Model file for the job. Use its own axes, mm. Face numbers are marked on the shaded views. A direction names the side the tool comes from. Give positions to 0.01 mm unless a question says otherwise; leave off trailing zeros. Write each loop counter-clockwise with the first axis right and the second up, starting at its lowest first coordinate (ties: lowest second). Pieces come first, ordered by that corner, then holes. Notation, with made-up numbers: (87.25, 26.5) - (116.25, 26.5) arc R18 cw to (116.25, 44.5) - close; hole circle Ø9 at (27.5, -33). An arc over 180 degrees is marked (long way). Use a Markdown table: item, result. Add a question column.
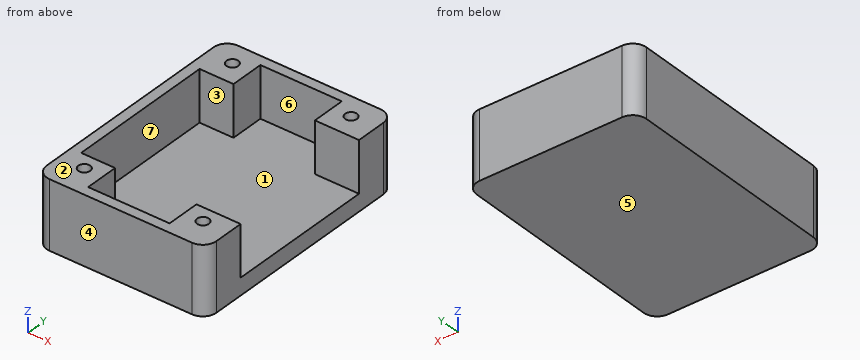
Autodesk Inventor part; units mm, degrees
ref_plane "YZ Plane" through (0, 0, 0) normal (1, 0, 0) x (0, 1, 0)
ref_plane "XZ Plane" through (0, 0, 0) normal (0, 1, 0) x (-1, 0, 0)
ref_plane "XY Plane" through (0, 0, 0) normal (0, 0, 1) x (1, 0, 0)
sketch "Sketch1" plane through (0, 0, 0) normal (0, 0, 1) x (1, 0, 0)
  line L0 (0, 0) -> (50, 0)
  line L1 (50, 0) -> (50, 70)
  line L2 (50, 70) -> (0, 70)
  line L3 (0, 70) -> (0, 0)
  dimension "d0" = 50
  dimension "d1" = 70
extrude "Extrusion1" add sketch "Sketch1" along normal blind 20
sketch "Sketch2" plane through (0, 0, 20) normal (0, 0, 1) x (1, 0, 0)
  line L0 (50, 70) -> (0, 70)
  line L1 (0, 0) -> (50, 0)
  line L2 (3, 67) -> (47, 67)
  line L3 (47, 67) -> (47, 3)
  line L4 (47, 3) -> (3, 3)
  line L5 (3, 3) -> (3, 67)
  line L6 (0, 70) -> (0, 0)
  dimension "d4" = 44
  dimension "d5" = 64
  dimension "d6" = 3
  dimension "d7" = 3
extrude "Extrusion2" cut sketch "Sketch2" against normal blind 15
sketch "Sketch3" plane through (0, 0, 20) normal (0, 0, 1) x (1, 0, 0)
  line L0 (50, 70) -> (0, 70)
  line L1 (0, 70) -> (13, 70)
  line L2 (13, 70) -> (13, 57)
  line L3 (13, 57) -> (0, 57)
  line L4 (0, 57) -> (0, 70)
  line L5 (0, 0) -> (50, 0)
  line L6 (0, 0) -> (13, 0)
  line L7 (13, 0) -> (13, 13)
  line L8 (13, 13) -> (0, 13)
  line L9 (0, 13) -> (0, 0)
  line L10 (50, 70) -> (37, 70)
  line L11 (37, 70) -> (37, 57)
  line L12 (37, 57) -> (50, 57)
  line L13 (50, 57) -> (50, 70)
  line L14 (50, 0) -> (37, 0)
  line L15 (37, 0) -> (37, 13)
  line L16 (37, 13) -> (50, 13)
  line L17 (50, 13) -> (50, 0)
  point P0 (37, 0)
  dimension "d10" = 13
  dimension "d11" = 13
extrude "Extrusion3" add sketch "Sketch3" against normal up to surface (15 mm away)
sketch "Sketch4" plane through (0, 0, 20) normal (0, 0, 1) x (1, 0, 0)
  line L0 (7.5, 63.5) -> (42.5, 63.5)
  line L1 (42.5, 63.5) -> (42.5, 8.5)
  line L2 (42.5, 8.5) -> (7.5, 8.5)
  line L3 (7.5, 8.5) -> (7.5, 63.5)
  circle A0 centre (7.5, 63.5) radius 1.75
  circle A1 centre (42.5, 63.5) radius 1.75
  circle A2 centre (42.5, 8.5) radius 1.75
  circle A3 centre (7.5, 8.5) radius 1.75
  line L4 (50, 70) -> (0, 70)
  line L5 (47, 57) -> (37, 57)
  line L6 (50, 0) -> (50, 70)
  point P0 (0, 0)
  dimension "d18" = 3.5
  dimension "d22" = 35
  dimension "d23" = 55
  dimension "d24" = 7.5
  dimension "d25" = 6.5
extrude "Extrusion4" cut sketch "Sketch4" against normal blind 5 contours L3 A0 L0 | L0 A0 L3 | A1 L1 L0 | L0 L1 A1 | A3 L2 L3 | L3 L2 A3 | A2 L1 L2 | L2 L1 A2
sketch "Sketch5" plane through (50, 0, 0) normal (1, 0, 0) x (0, 0, -1)
  line L0 (-20, 13) -> (-5, 13)
  line L1 (-20, 57) -> (-5, 57)
  line L2 (-5, 13) -> (-5, 57)
  line L3 (-20, 13) -> (-5, 13)
  line L4 (-5, 13) -> (-5, 57)
  line L5 (-5, 57) -> (-20, 57)
  line L6 (-20, 57) -> (-20, 13)
  point P0 (0, 0)
extrude "Extrusion5" cut sketch "Sketch5" against normal up to surface (47 mm away)
fillet "Fillet2" radius 4 4 edges at (0, 70, 10) (50, 70, 10) (50, 0, 10) (0, 0, 10)
properties part number "HOLDER"
(1) Flat gauge pins, fed straight in: pin 1 (1.5 mm diameter, centred on x = 9, y = 39.5, fed in from +Z); pin 2 (3 mm diameter, centred on x = 7.5, y = 8.5, fed in from +Z); pin 3 (7.5 mm diameter, centred on y = 37.5, z = 15, fed in from +X). Where does each tip first touch, or does it go through?
(2) Band-saw the part on A-A (z = 17.5). Write the cut outline in (x, y).
(3) Which spindle directions (+Z, -Z, +X, -X, +Y, -Y) get a long thin tool onto all of the face, cutting with end or side? Do the marked faces 5, 6 and 7. Say none if no direction does.
(4) Band-saw the part on B-B (y = 12). Write the cut outline in (x, z).
(5) Probe probe 1 along Y at (x, z) = (7.5, 16.05); probe 2 along X at (y, z) = (8.5, 18.65); probe 3 along Y at (x, z) = (45, 7). List the from-to ranges inside material, lowest first. Write a range as [from, to].
(6) Two-plate mould, pull along Y, no slides. Class the marked faces 1, 2, 3 and 4: +Y half, -Y half, draft (parallel to the pull), parting line (faces both ways), or undercut.
(7) Band-saw the part on C-C (z = 7). Write the cut outline in (x, y).
(8) Band-saw the part on D-D (x = 25.5). Write the cut outline in (y, z).
Model answer:
| question | item | result |
|---|---|---|
| 1 | pin 1 | stops at z = 5 |
| 1 | pin 2 | stops at z = 15 |
| 1 | pin 3 | stops at x = 3 |
| 2 | outline | (0, 4) arc R4 ccw to (4, 0) - (46, 0) arc R4 ccw to (50, 4) - (50, 13) - (37, 13) - (37, 3) - (13, 3) - (13, 13) - (3, 13) - (3, 57) - (13, 57) - (13, 67) - (37, 67) - (37, 57) - (50, 57) - (50, 66) arc R4 ccw to (46, 70) - (4, 70) arc R4 ccw to (0, 66) - close; hole circle Ø3.5 at (7.5, 8.5); hole circle Ø3.5 at (7.5, 63.5); hole circle Ø3.5 at (42.5, 8.5); hole circle Ø3.5 at (42.5, 63.5) |
| 3 | face 5 | -Z, +X, -X, +Y, -Y |
| 3 | face 6 | +Z |
| 3 | face 7 | +Z, +X |
| 4 | outline | (0, 0) - (50, 0) - (50, 20) - (37, 20) - (37, 5) - (13, 5) - (13, 20) - (0, 20) - close |
| 5 | probe 1 | y = [0, 6.75], [10.25, 13], [57, 61.75], [65.25, 70] |
| 5 | probe 2 | x = [0, 5.75], [9.25, 13], [37, 40.75], [44.25, 50] |
| 5 | probe 3 | y = [0, 13], [57, 70] |
| 6 | face 1 | undercut |
| 6 | face 2 | draft |
| 6 | face 3 | undercut |
| 6 | face 4 | -Y half |
| 7 | outline | (0, 4) arc R4 ccw to (4, 0) - (46, 0) arc R4 ccw to (50, 4) - (50, 13) - (37, 13) - (37, 3) - (13, 3) - (13, 13) - (3, 13) - (3, 57) - (13, 57) - (13, 67) - (37, 67) - (37, 57) - (50, 57) - (50, 66) arc R4 ccw to (46, 70) - (4, 70) arc R4 ccw to (0, 66) - close |
| 8 | outline | (0, 0) - (70, 0) - (70, 20) - (67, 20) - (67, 5) - (3, 5) - (3, 20) - (0, 20) - close |
